Design review of the part built by this model. Coordinates are the model's own, in mm. Face numbers are marked on the shaded views. A direction names the side the tool comes from. Give positions to 0.01 mm unless a question says otherwise; leave off trailing zeros. Write each loop counter-clockwise with the first axis right and the second up, starting at its lowest first coordinate (ties: lowest second). Pieces come first, ordered by that corner, then holes. Notation, with made-up numbers: M 55.5,32.25 L 86.5,32.25 A14 ccw 86.5,45.25 Z; hole C 48,9 d2. An arc over 180 degrees is marked long. Use one line per item in the form item = value. Start each with the question number.
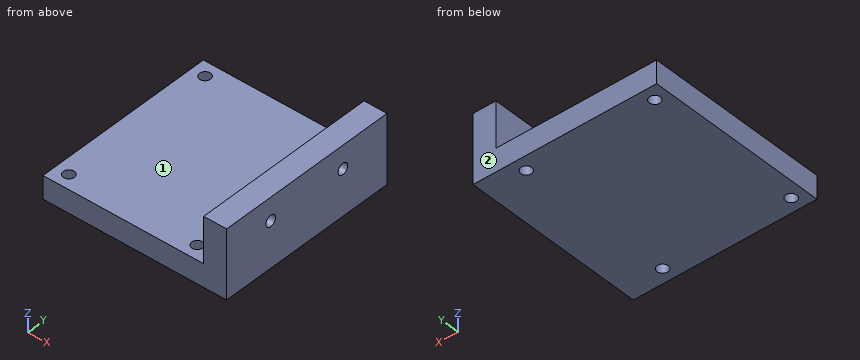
from build123d import *

# Parameters (mm, degrees)
F0_W     = 40
F0_H     = 40
F1_DEPTH = 5
F2_W     = 5
F2_H     = 40
F3_DEPTH = 10
F5_D     = 2.4
F7_D     = 2.4


with BuildPart() as f1:
    # F0 (on Top) → F1 (new body)
    with BuildSketch(Plane.XY):
        Rectangle(F0_W, F0_H)
    extrude(amount=F1_DEPTH)

    # F2 (on face) → F3 (join)
    with BuildSketch(Plane.XY.offset(5)):
        with Locations((17.5, 0)):
            Rectangle(F2_W, F2_H)
    extrude(amount=F3_DEPTH)

    # F5 (through all)
    with Locations(Plane.YZ.offset(20)):
        with Locations((-9, 10), (9, 10)):
            Hole(F5_D / 2)

    # F7 (through all)
    with Locations(Plane.XY.offset(5)):
        with Locations((-17, 17), (11, 17), (11, -17), (-17, -17)):
            Hole(F7_D / 2)


solid = f1.part
1. We need section A-A (y = -17). State the section outline as (x, z) points, and give its area (3 significant figures).
2. Clearance check with flat-ended pins moving along their axes: pin 1 Ø5 at (y, z) = (-2.5, 10.5) entering from -X; pin 2 Ø3 at (x, y) = (-17, -17) entering from +Z; pin 3 Ø3 at (y, z) = (9, 10) entering from +X. State where each tip first meets the part, or that it passes through.
3. We need section C-C (z = 10). State the section outline as (x, y) points, and give its area (3 significant figures).
4. We need section B-B (x = -17). State the section outline as (y, z) points, and give its area (3 significant figures).
5. We need section D-D (y = 11). State the section outline as (x, z) points, and give its area (3 significant figures).
6. To check wall thickness, follow L1, parallel to Y at x = -17, z = 1.4; L2, parallel to Z at x = 16, y = -9; L3, parallel to Z at x = 12.5, y = 15. State the ranges of each line that lie inside material, in increasing order.
7. For the marked faces 1 and 2, list the 3-axis set-ups (+Z, -Z, +X, -X, +Y, -Y) from which the entire face can be reached by the end or side of a thin tool; tool diameter is ignored.
Answer block:
q1.outline = M -20,0 L -18.2,0 L -18.2,5 L -20,5 Z; M -15.8,0 L 9.8,0 L 9.8,5 L -15.8,5 Z; M 12.2,0 L 20,0 L 20,15 L 15,15 L 15,5 L 12.2,5 Z
q1.area = 226 mm^2
q2.pin_1 = 15
q2.pin_2 = 5
q2.pin_3 = 20
q3.outline = M 15,-20 L 20,-20 L 20,-10.2 L 15,-10.2 Z; M 15,-7.8 L 20,-7.8 L 20,7.8 L 15,7.8 Z; M 15,10.2 L 20,10.2 L 20,20 L 15,20 Z
q3.area = 176 mm^2
q4.outline = M -20,0 L -18.2,0 L -18.2,5 L -20,5 Z; M -15.8,0 L 15.8,0 L 15.8,5 L -15.8,5 Z; M 18.2,0 L 20,0 L 20,5 L 18.2,5 Z
q4.area = 176 mm^2
q5.outline = M -20,0 L 20,0 L 20,15 L 15,15 L 15,5 L -20,5 Z
q5.area = 250 mm^2
q6.L1 = -20 to -18.2, -15.8 to 15.8, 18.2 to 20
q6.L2 = 0 to 8.8, 11.2 to 15
q6.L3 = 0 to 5
q7.face_1 = +Z, -X, +Y, -Y
q7.face_2 = +Z, -Z, +X, -X, +Y
